Autodesk Fusion 360 part; units mm, degrees
sketch "Sketch1" plane through (0, 0, 0) normal (0, 0, 1) x (1, 0, 0)
  line L0 (75, 75) -> (-75, 75)
  line L1 (-75, 75) -> (-75, -75)
  line L2 (-75, -75) -> (75, -75)
  line L3 (75, -75) -> (75, 75)
  line L4 (75, 75) -> (-75, -75) construction
  line L5 (-75, 75) -> (75, -75) construction
  line L6 (60, 60) -> (-60, 60)
  line L7 (-60, 60) -> (-60, -60)
  line L8 (-60, -60) -> (60, -60)
  line L9 (60, -60) -> (60, 60)
  line L10 (60, 60) -> (-60, -60) construction
  line L11 (-60, 60) -> (60, -60) construction
  dimension "d1" = 150
  dimension "d2" = 150
  dimension "d3" = 120
  dimension "d4" = 120
extrude "Extrude1" add sketch "Sketch1" along normal blind 10 contours L6 L7 L8 L9
extrude "Extrude2" add sketch "Sketch1" along normal blind 150
fillet "Fillet1" radius 2 12 edges at (-60, 0, 150) (0, 60, 150) (60, 0, 150) (0, -60, 150) (0, 60, 10) (-60, 0, 10) (-60, 60, 80) (0, -60, 10) (-60, -60, 80) (60, -60, 80) (60, 0, 10) (60, 60, 80)
fillet "Fillet2" radius 4 4 edges at (75, -75, 75) (-75, -75, 75) (75, 75, 75) (-75, 75, 75)
fillet "Fillet3" radius 2 8 edges at (-73.8284, 73.8284, 150) (-75, 0, 150) (-73.8284, -73.8284, 150) (0, -75, 150) (73.8284, -73.8284, 150) (75, 0, 150) (73.8284, 73.8284, 150) (0, 75, 150)
Model file for the job. Use its own axes, mm. A direction names the side the tool comes from. Coordinates: 2 decimals unless noted, no trailing zeros. Write each loop counter-clockwise with the first axis right and the second up, starting at its lowest first coordinate (ties: lowest second). Pieces come first, ordered by that corner, then holes. Notation, with made-up numbers: (71.5, -21) - (125.5, -21) arc R12 ccw to (125.5, -17) - close; hole circle Ø4 at (-9, 51.5). An arc over 180 degrees is marked (long way). Use a Markdown table: item, result. Add a question column.
Item 1: Band-saw the part on A-A, the plane z = 128.5. Write the cut outline in (x, y), and give its area (3 significant figures).
Item 2: Band-saw the part on B-B, the plane y = -47. Write the cut outline in (x, z), and give its area (3 significant figures).
Item 3: Two-plate mould, pull along X, no slides. Class faces 3 (the face through (1, 75, 73)), 4 (the face through (-1, 1, 10)), 5 (the face through (75, -1, 73)): pulls with the +X half, pulls with the -X half, needs draft (parallel to the pull), parting line crosses it, or undercut.
Item 4: Drop a flat-ended pin along its axis: pin 1 (1.5 mm diameter, centred on x = -44, y = 55.5, fed in from +Z). Give the stop position or say it passes through.
Item 5: 3-axis set-ups, long thin cutter, end or side, ignore diameter. For faces 1 (the face through (-1, -75, 73)), 2 (the face through (60, -1, 79)): which of +Z, -Z, +X, -X, +Y, -Y reach the whole face in a straight line?
Item 6: Drill centre lines: line 1 along Y through (x, z) = (17.5, 24); line 2 along Z through (x, y) = (-6, -46.5). Where is each one in solid material? Low to high.
A:
| question | item | result |
|---|---|---|
| 1 | outline | (-75, -71) arc R4 ccw to (-71, -75) - (71, -75) arc R4 ccw to (75, -71) - (75, 71) arc R4 ccw to (71, 75) - (-71, 75) arc R4 ccw to (-75, 71) - close; hole (-60, -58) arc R2 ccw to (-58, -60) - (58, -60) arc R2 ccw to (60, -58) - (60, 58) arc R2 ccw to (58, 60) - (-58, 60) arc R2 ccw to (-60, 58) - close |
| 1 | area | 8,090 mm² |
| 2 | outline | (-75, 0) - (75, 0) - (75, 148) arc R2 ccw to (73, 150) - (62, 150) arc R2 ccw to (60, 148) - (60, 12) arc R2 cw to (58, 10) - (-58, 10) arc R2 cw to (-60, 12) - (-60, 148) arc R2 ccw to (-62, 150) - (-73, 150) arc R2 ccw to (-75, 148) - close |
| 2 | area | 5,700 mm² |
| 3 | face 3 | needs draft |
| 3 | face 4 | undercut |
| 3 | face 5 | pulls with the +X half |
| 4 | pin 1 | stops at z = 10 |
| 5 | face 1 | +Z, -Z, +X, -X, -Y |
| 5 | face 2 | +Z |
| 6 | line 1 | y = -75 to -60, 60 to 75 |
| 6 | line 2 | z = 0 to 10 |
